Part print with two shaded views. Sizes in mm from the minimum x, y, z corner. Round coordinates to 2 decimals unless told otherwise and drop trailing zeros. Order: outer loops, then holes, each group sorted by start corner. A loop starts at its lowest first (then second) coordinate and runs counter-clockwise, first axis right, second up. Notation, with made-up numbers: (1, 52) -> (20, 52) arc R27 cw to (20, 76) -> close; hole circle Ø11 at (14.5, -11.75). An arc over 180 degrees is marked (long way). Answer as a JSON object with one key per item and string values.
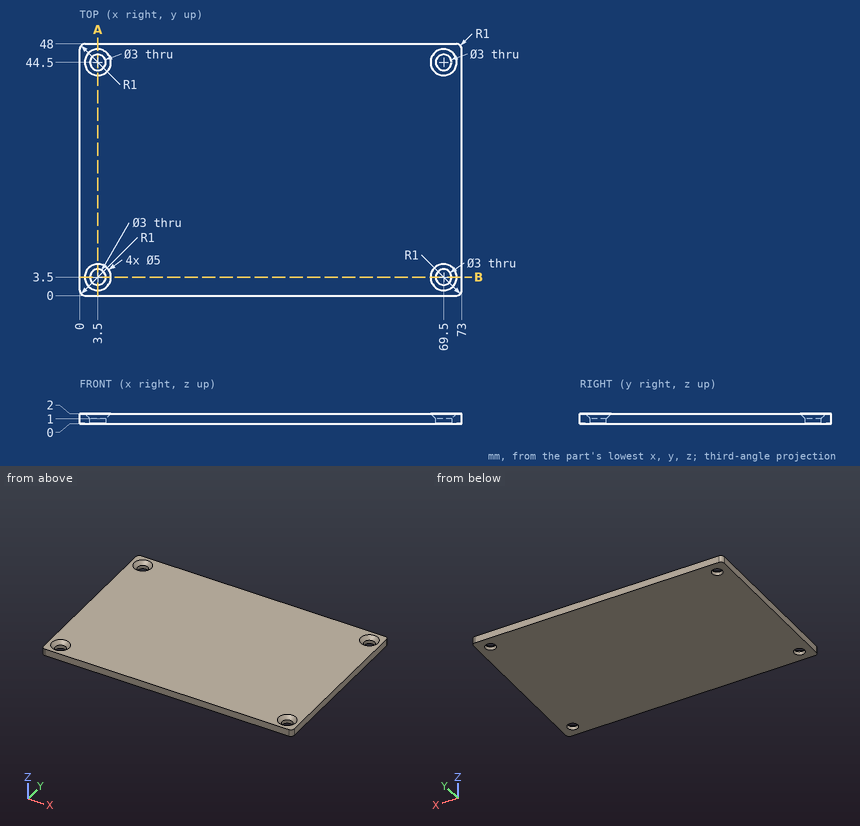
1) Probe L1, parallel to Y at x = 69.5, z = 0.75; L2, parallel to Y at x = 3.5, z = 1.85; L3, parallel to X at y = 43.5, z = 0.85. List the from-to ranges inside material, lowest first. Write a range as from..to.
Checked values:
{"L1": "y = 0..2, 5..43, 46..48", "L2": "y = 0..1.15, 5.85..42.15, 46.85..48", "L3": "x = 0..2.38, 4.62..68.38, 70.62..73"}
2) Cut at B-B, the plane y = 3.5. Give the cut face in (x, z), plus the area to 3 significant figures.
Checked values:
{"outline": "(0, 0) -> (2, 0) -> (2, 1) -> (1, 2) -> (0, 2) -> close; (5, 0) -> (68, 0) -> (68, 1) -> (67, 2) -> (6, 2) -> (5, 1) -> close; (71, 0) -> (73, 0) -> (73, 2) -> (72, 2) -> (71, 1) -> close", "area": "132 mm²"}
3) Cut at A-A, the plane x = 3.5. Give the cut face in (y, z).
Checked values:
{"outline": "(0, 0) -> (2, 0) -> (2, 1) -> (1, 2) -> (0, 2) -> close; (5, 0) -> (43, 0) -> (43, 1) -> (42, 2) -> (6, 2) -> (5, 1) -> close; (46, 0) -> (48, 0) -> (48, 2) -> (47, 2) -> (46, 1) -> close"}
4) Flat gauge pin, fed straight in: pin 1 Ø2.5 at (x, y) = (69.5, 44.5) entering from +Z. Where does the tip first touch, or does it go through?
Checked values:
{"pin 1": "passes through"}
